Could you check a few things on this model? Use its own coordinates, in mm. A direction names the side the tool comes from. Coordinates: 2 decimals unless noted, no trailing zeros. Order: outer loops, then holes, each group sorted by start corner. A loop starts at its lowest first (then second) coordinate and runs counter-clockwise, first axis right, second up. Notation, with made-up numbers: (-10.5, 72.5) -> (39.5, 72.5) arc R16 cw to (39.5, 97.5) -> close; hole circle Ø3 at (84.5, 47). An arc over 180 degrees is marked (long way). Use a Markdown table: item, result. Add a question column.
1) Thinking about a two-plate mould opening in Y: for faces 1 (the flat face through (-38, -34.309, 2)), 2 (the flat face through (-10.742, -45, 2)), 3 (the flat face through (-55, -77.145, 2)), which applies, +Y half, -Y half, draft (parallel to the pull), parting line (faces both ways), or undercut?
2) If we section it at D-D (y = -36): Write out the boundary of the cut face in (x, z) (3 decimals), plus the area to 3 significant figures.
3) If we section it at C-C (z = 1): Give the number of separate pieces and of enclosed holes in the cut face, plus the area to 3 significant figures.
4) Which directions (+Z, -Z, +X, -X, +Y, -Y) give clear straight access to the entire face, cutting with the end or side of a thin tool? Please do faces 4 (the flat face through (-56, -45, 0)), 5 (the flat face through (-48, -69.339, 2)).
5) If we section it at B-B (x = -39): Write out the boundary of the cut face in (y, z) (3 decimals).
6) If we section it at A-A (y = -65): Write out the boundary of the cut face in (x, z) (3 decimals), plus the area to 3 significant figures.
7) If I drill on L1, parallel to X at y = -31, z = 0.4; L2, parallel to X at y = -32.5, z = 1.45; L3, parallel to Y at x = -48, z = 1.15, over which ranges is the centre line in solid material (lowest first)? Write a range as [from, to].
Autodesk Inventor part; units mm, degrees
ref_plane "YZ Plane" through (0, 0, 0) normal (1, 0, 0) x (0, 1, 0)
ref_plane "XZ Plane" through (0, 0, 0) normal (0, 1, 0) x (-1, 0, 0)
ref_plane "XY Plane" through (0, 0, 0) normal (0, 0, 1) x (1, 0, 0)
sketch "Sketch1" plane through (0, 0, 0) normal (0, 0, 1) x (1, 0, 0)
  line L0 (-99.6423, -13.6452) -> (-10.7423, -13.6452)
  line L1 (-10.7423, -13.6452) -> (-10.7423, -77.1452)
  line L2 (-10.7423, -77.1452) -> (-99.6423, -77.1452)
  line L3 (-99.6423, -77.1452) -> (-99.6423, -13.6452)
  point P0 (0, 0)
  dimension "d0" = 88.9
  dimension "d1" = 63.5
extrude "Extrusion1" add sketch "Sketch1" along normal blind 3.175
sketch "Sketch2" plane through (0, 0, 3.175) normal (0, 0, 1) x (1, 0, 0)
  line L0 (-99.6423, -77.1452) -> (-10.7423, -77.1452)
  line L1 (-10.7423, -13.6452) -> (-99.6423, -13.6452)
  circle A0 centre (-59.962, -31.2669) radius 10.3124 construction
  arc A1 (-56.7195, -38.3027) -> (-63.2044, -38.3027) centre (-59.962, -31.2669) ccw
  circle A2 centre (-69.0552, -48.9507) radius 9.0932 construction
  arc A3 (-66.3161, -53.6751) -> (-71.7943, -53.6751) centre (-69.0552, -48.9507) ccw
  circle A4 centre (-40.9053, -48.9507) radius 5.2451 construction
  circle A5 centre (-40.9053, -48.9507) radius 2.9464
  line L2 (-63.2044, -38.3027) -> (-56.7195, -38.3027)
  line L3 (-71.7943, -53.6751) -> (-66.3161, -53.6751)
  circle A6 centre (-38.1662, -29.5849) radius 9.0932 construction
  arc A7 (-35.4272, -34.3093) -> (-40.9053, -34.3093) centre (-38.1662, -29.5849) ccw
  line L4 (-40.9053, -34.3093) -> (-35.4272, -34.3093)
  arc A8 (-85.4364, -48.1452) -> (-88.9005, -48.1452) centre (-87.1685, -45.3952) ccw
  line L5 (-85.4364, -48.1452) -> (-88.9005, -48.1452)
  circle A9 centre (-87.1685, -45.3952) radius 5.5 construction
  arc A10 (-64.584, -70.0116) -> (-68.0481, -70.0116) centre (-66.3161, -67.2616) ccw
  line L6 (-64.584, -70.0116) -> (-68.0481, -70.0116)
  circle A11 centre (-66.3161, -67.2616) radius 5.5 construction
  arc A12 (-46.6132, -69.3388) -> (-50.0773, -69.3388) centre (-48.3452, -66.5888) ccw
  line L7 (-46.6132, -69.3388) -> (-50.0773, -69.3388)
  circle A13 centre (-48.3452, -66.5888) radius 5.5 construction
  arc A14 (-20.5575, -48.0295) -> (-24.0216, -48.0295) centre (-22.2896, -45.2795) ccw
  line L8 (-20.5575, -48.0295) -> (-24.0216, -48.0295)
  circle A15 centre (-22.2896, -45.2795) radius 5.5 construction
  point P0 (0, 0)
  dimension "d18" = 20.6248
  dimension "d19" = 15.494
  dimension "d20" = 18.1864
  dimension "d21" = 10.922
  dimension "d22" = 10.4902
  dimension "d23" = 5.8928
  dimension "d24" = 7.0358
  dimension "d25" = 4.7244
  dimension "d26" = 18.1864
  dimension "d27" = 10.922
  dimension "d28" = 4.7244
  dimension "d32" = 28.1945
  dimension "d36" = 6.5
  dimension "d37" = 2.75
  dimension "d38" = 11
  dimension "d39" = 6.5
  dimension "d40" = 2.75
  dimension "d41" = 11
  dimension "d42" = 6.5
  dimension "d43" = 2.75
  dimension "d44" = 11
  dimension "d45" = 6.5
  dimension "d46" = 2.75
  dimension "d47" = 11
extrude "Extrusion2" cut sketch "Sketch2" against normal blind 6.35
properties part number "DishFront_BackPlate"
Answer sheet:
| question | item | result |
|---|---|---|
| 1 | face 1 | undercut |
| 1 | face 2 | draft |
| 1 | face 3 | -Y half |
| 2 | outline | (-99.642, 0) -> (-66.095, 0) -> (-66.095, 3.175) -> (-99.642, 3.175) -> close; (-53.829, 0) -> (-10.742, 0) -> (-10.742, 3.175) -> (-53.829, 3.175) -> close |
| 2 | area | 243 mm2 |
| 3 | separate pieces | 1 |
| 3 | enclosed holes | 8 |
| 3 | area | 5,120 mm2 |
| 4 | face 4 | -Z, +X, -X, +Y, -Y |
| 4 | face 5 | +Z, -Z |
| 5 | outline | (-77.145, 0) -> (-51.198, 0) -> (-51.198, 3.175) -> (-77.145, 3.175) -> close; (-46.703, 0) -> (-34.309, 0) -> (-34.309, 3.175) -> (-46.703, 3.175) -> close; (-24.188, 0) -> (-13.645, 0) -> (-13.645, 3.175) -> (-24.188, 3.175) -> close |
| 6 | outline | (-99.642, 0) -> (-68.65, 0) -> (-68.65, 3.175) -> (-99.642, 3.175) -> close; (-63.982, 0) -> (-51.18, 0) -> (-51.18, 3.175) -> (-63.982, 3.175) -> close; (-45.51, 0) -> (-10.742, 0) -> (-10.742, 3.175) -> (-45.51, 3.175) -> close |
| 6 | area | 249 mm2 |
| 7 | L1 | [-99.64, -67.7], [-52.22, -43.44], [-32.89, -10.74] |
| 7 | L2 | [-99.64, -67.61], [-52.31, -42.78], [-33.55, -10.74] |
| 7 | L3 | [-77.15, -69.34], [-63.36, -13.65] |
